Geometry: final body of the model. Coordinates: model frame, mm. Give positions to 0.01 mm unless a question says otherwise; leave off trailing zeros. Order: outer loops, then holes, each group sorted by start corner. A loop starts at its lowest first (then second) coordinate and runs counter-clockwise, first axis right, second up. Notation, with made-up numbers: (27, 30) -> (82, 30) arc R16 ccw to (82, 59) -> close; hole circle Ø1 at (-31, -15.5). An arc over 180 degrees is marked (long way). Write item = value, one per line.
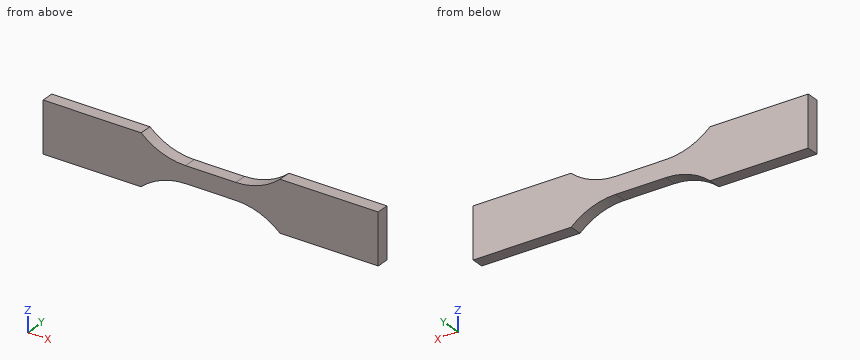
```python
from build123d import *

# Parameters (mm, degrees)
BOSS_EXTRUDE1_DEPTH                      = 2.385
MIRROR1_AT_THE_SECOND_PLANE_COPY_1_DEPTH = 2.385
SCALE1_SCALE                             = 0.3144


with BuildPart() as part:
    # Sketch1 → Boss-Extrude1 (new body)
    with BuildSketch(Plane(origin=(0, 0, 0), x_dir=(1, 0, 0), z_dir=(0, 1, 0))):
        with BuildLine():
            Line((0, 1.59), (4.765, 1.59))
            ThreePointArc((4.765, 1.59), (9.255128061, 2.410237797), (13.165260413, 4.765))
            Line((13.165260413, 4.765), (31.75, 4.765))
            Line((31.75, 4.765), (31.75, 0))
            Line((31.75, 0), (0, 0))
            Line((0, 0), (0, 1.59))
        make_face()
    boss_extrude1 = extrude(amount=BOSS_EXTRUDE1_DEPTH)



with BuildPart() as mirror1_1:
    # Mirror1: Boss-Extrude1 across plane
    add(boss_extrude1.mirror(Plane(origin=(0, 0, 0), x_dir=(0, 0, 1), z_dir=(1, 0, 0))))


with BuildPart() as part_1:
    add(part.part)

    add(mirror1_1.part)  # Mirror1 at the second plane merges Mirror1_1
    # Mirror1 at the second plane: Boss-Extrude1 across plane
    add(boss_extrude1.mirror(Plane.XY))

    # Mirror1 at the second plane copy 1 sketc → Mirror1 at the second plane copy 1 (add)
    with BuildSketch(Plane(origin=(0, 0, 0), x_dir=(-1, 0, 0), z_dir=(0, 1, 0))):
        with BuildLine():
            Line((0, 1.59), (4.765, 1.59))
            ThreePointArc((4.765, 1.59), (9.255128061, 2.410237797), (13.165260413, 4.765))
            Line((13.165260413, 4.765), (31.75, 4.765))
            Line((31.75, 4.765), (31.75, 0))
            Line((31.75, 0), (0, 0))
            Line((0, 0), (0, 1.59))
        make_face()
    extrude(amount=MIRROR1_AT_THE_SECOND_PLANE_COPY_1_DEPTH)


with BuildPart() as part_2:
    # Scale1: scaled about (0, 1.1925, 0)
    add(part_1.part.scale(SCALE1_SCALE).moved(Location((0, 0.817578, 0))))


solid = part_2.part
```
1) Section query C-C (z = 1.1). Output: boundary loops of the cut face in (x, y), plus the area to 3 significant figures.
Check sheet entries:
outline = (-9.98, 0.82) -> (-3.6, 0.82) -> (-3.6, 1.57) -> (-9.98, 1.57) -> close; (3.6, 0.82) -> (9.98, 0.82) -> (9.98, 1.57) -> (3.6, 1.57) -> close
area = 9.57 mm²
2) Section query A-A (z = -1.15). Output: boundary loops of the cut face in (x, y).
Check sheet entries:
outline = (-9.98, 0.82) -> (-3.68, 0.82) -> (-3.68, 1.57) -> (-9.98, 1.57) -> close; (3.68, 0.82) -> (9.98, 0.82) -> (9.98, 1.57) -> (3.68, 1.57) -> close
3) Line query: line 1 (Z direction, x = 1, y = 1.3); line 2 (X direction, y = 0.85, z = 1.05); line 3 (X direction, y = 1.05, z = 0.8). Output: solid intervals per line, ascending. Write a range as from..to.
Check sheet entries:
line_1 = -0.5..0.5
line_2 = -9.98..-3.52, 3.52..9.98
line_3 = -9.98..-3.02, 3.02..9.98
4) Section query B-B (y = 1.25). Output: boundary loops of the cut face in (x, z), plus the area to 3 significant figures.
Check sheet entries:
outline = (-9.98, -1.5) -> (-4.14, -1.5) arc R3.99 cw to (-1.5, -0.5) -> (1.5, -0.5) arc R3.99 cw to (4.14, -1.5) -> (9.98, -1.5) -> (9.98, 1.5) -> (4.14, 1.5) arc R3.99 cw to (1.5, 0.5) -> (-1.5, 0.5) arc R3.99 cw to (-4.14, 1.5) -> (-9.98, 1.5) -> close
area = 46.6 mm²
5) Section query D-D (x = -3). Output: boundary loops of the cut face in (y, z), plus the area to 3 significant figures.
Check sheet entries:
outline = (0.82, -0.79) -> (1.57, -0.79) -> (1.57, 0.79) -> (0.82, 0.79) -> close
area = 1.19 mm²
